The figure shows three views and two pictorial views of one solid part (mm, origin at its lowest corner). Answer the questions. A direction names the side the tool comes from. Coordinates: 2 decimals unless noted, no trailing zeros. Write each loop counter-clockwise with the first axis right and the second up, starting at its lowest first coordinate (ties: lowest second). Pieces come first, ordered by that corner, then holes. Notation, with made-up numbers: (83.25, 75.25) - (93.25, 75.25) arc R33 ccw to (93.25, 104.25) - close; hole circle Ø9 at (-22.5, 4). An arc over 180 degrees is marked (long way). Use a Markdown table: item, result. Add a question column.
(1) A tool of negligible diameter and unlimited length cuts with its end or side. For the marked faces 5 and 6, from which of +Z, -Z, +X, -X, +Y, -Y can it reach the whole face along a straight path? Write none if from no direction.
(2) The part is cut by section D-D, the plane z = 28.5. Give the vertices of the cut face in (x, y), then the cut area to 3 significant figures.
(3) The part is cut by section B-B, the plane z = 15. Give the vertices of the cut face in (x, y), then the cut area to 3 significant figures.
(4) Given pin 1 Ø12 at (x, y) = (32.5, 20) entering from -Z; pin 2 Ø4 at (y, z) = (12, 50) entering from +X, each flat-ended and moving along its own axis, determine where each tip first touches the part or whether it passes through.
(5) Find the intervals of material crossed by line 1 (Y direction, x = 3.25, z = 15); line 2 (X direction, y = 4.25, z = 46); line 3 (Z direction, x = 27.5, y = 8), in increasing order. Write a range as from..to.
(6) The part is cut by section A-A, the plane y = 15. Give the vertices of the cut face in (x, z), then the cut area to 3 significant figures.
(7) The part is cut by section C-C, the plane x = 45.5. Give the vertices of the cut face in (y, z).
(8) For a pull along Z with two mould halves and no side action, classify the marked faces 1, 2, 3 and 4 as released by +Z, released by -Z, zero draft, split by the parting line, or undercut.
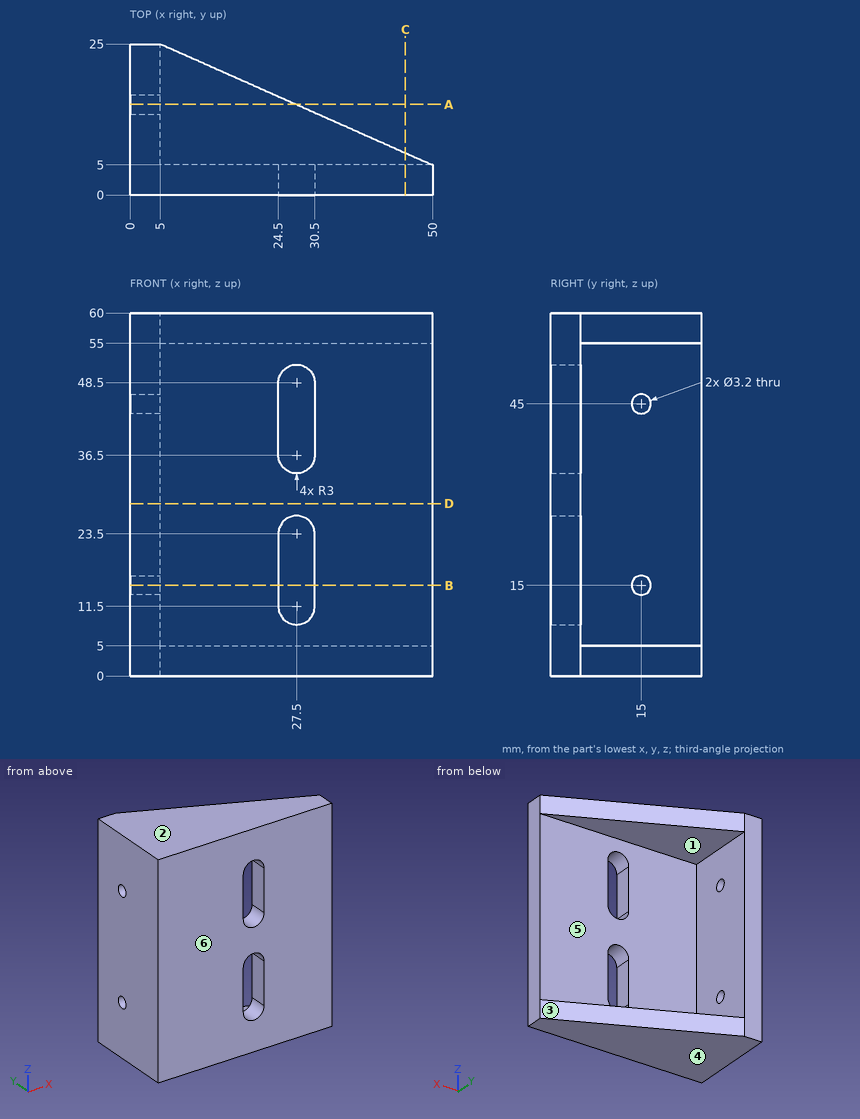
Model answer:
| question | item | result |
|---|---|---|
| 1 | face 5 | +X, +Y |
| 1 | face 6 | +Z, -Z, +X, -X, -Y |
| 2 | outline | (0, 0) - (50, 0) - (50, 5) - (5, 5) - (5, 25) - (0, 25) - close |
| 2 | area | 350 mm^2 |
| 3 | outline | (0, 0) - (24.5, 0) - (24.5, 5) - (5, 5) - (5, 13.4) - (0, 13.4) - close; (0, 16.6) - (5, 16.6) - (5, 25) - (0, 25) - close; (30.5, 0) - (50, 0) - (50, 5) - (30.5, 5) - close |
| 3 | area | 304 mm^2 |
| 4 | pin 1 | through |
| 4 | pin 2 | x = 5 |
| 5 | line 1 | 0..13.4, 16.6..25 |
| 5 | line 2 | 0..24.5, 30.5..50 |
| 5 | line 3 | 0..5, 55..60 |
| 6 | outline | (0, 0) - (27.5, 0) - (27.5, 5) - (5, 5) - (5, 13.4) - (0, 13.4) - close; (0, 16.6) - (5, 16.6) - (5, 43.4) - (0, 43.4) - close; (0, 46.6) - (5, 46.6) - (5, 55) - (27.5, 55) - (27.5, 60) - (0, 60) - close |
| 6 | area | 493 mm^2 |
| 7 | outline | (0, 0) - (7, 0) - (7, 5) - (5, 5) - (5, 55) - (7, 55) - (7, 60) - (0, 60) - close |
| 8 | face 1 | undercut |
| 8 | face 2 | released by +Z |
| 8 | face 3 | zero draft |
| 8 | face 4 | released by -Z |
